```python
from build123d import *

# Parameters (mm, degrees)
HOLE_WIZARD_M3_1_D     = 2.5
HOLE_WIZARD_M3_1_DEPTH = 10
HOLE_WIZARD_M3_2_D     = 2.5
HOLE_WIZARD_M3_2_DEPTH = 9.5
HOLE_WIZARD_M3_2_TIP   = 0.751075774
EXTRUDE_START          = 6
SKETCH_9_R             = 3.5
SKETCH_9_R_2           = 3
EXTRUDE_1_DEPTH        = 6


with BuildPart() as part:
    # 草图1 → 旋转1 (revolve)
    with BuildSketch(Plane.XY, mode=Mode.PRIVATE) as revolve_1_sk:
        Polygon((0, 9), (0, 3), (57.5, 3), (57.5, 8.75), (41.5, 8.75), (41.5, 9), (36.5, 9), (36.5, 6), (10, 6), (10, 9), align=None)
    revolve(revolve_1_sk.sketch.rotate(Axis((0, 0, 0), (1, 0, 0)), 90), axis=Axis((0, 0, 0), (1, 0, 0)))

    # M3 螺纹孔1
    with Locations(Plane.ZY):
        with Locations((0, 6), (6, 0), (0, -6), (-6, 0)):
            Hole(HOLE_WIZARD_M3_1_D / 2, depth=HOLE_WIZARD_M3_1_DEPTH)

    # M3 螺纹孔2
    with Locations(Plane(origin=(57.5, 0, 0), x_dir=(0, 0, -1), z_dir=(1, 0, 0))):
        with Locations((0, 6.25), (6.25, 0), (0, -6.25), (-6.25, 0)):
            Hole(HOLE_WIZARD_M3_2_D / 2, depth=HOLE_WIZARD_M3_2_DEPTH)
            with Locations((0, 0, -(HOLE_WIZARD_M3_2_DEPTH + HOLE_WIZARD_M3_2_TIP / 2))):  # 118° drill point
                Cone(0, HOLE_WIZARD_M3_2_D / 2, HOLE_WIZARD_M3_2_TIP, mode=Mode.SUBTRACT)

    # 草图9 → 凸台-拉伸1 (add)
    with BuildSketch(Plane(origin=(57.5, 0, 0), x_dir=(0, 0, -1), z_dir=(1, 0, 0)).offset(EXTRUDE_START)):
        with Locations(Location((0, 0, 0), (0, 0, 180))):
            Circle(SKETCH_9_R)
        with Locations(Location((0, 0, 0), (0, 0, 180))):
            Circle(SKETCH_9_R_2, mode=Mode.SUBTRACT)
    extrude(amount=-EXTRUDE_1_DEPTH)


solid = part.part
```
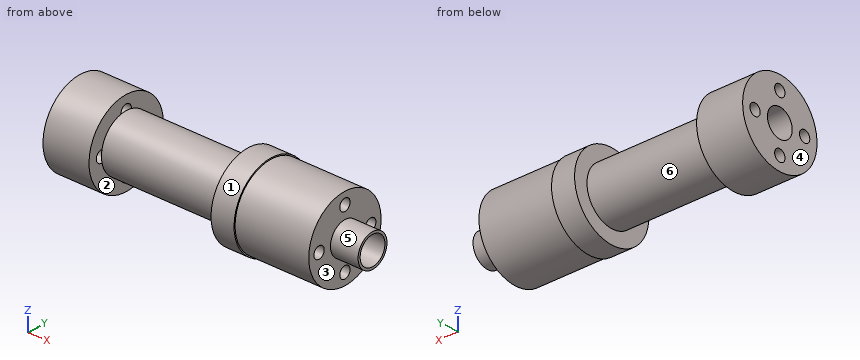
Input: part model. Units: mm. Frame: model coordinates. Face numbers are marked on the shaded views. A direction names the side the tool comes from. Give positions to 0.01 mm unless a question says otherwise; leave off trailing zeros. Order: outer loops, then holes, each group sorted by start corner. A loop starts at its lowest first (then second) coordinate and runs counter-clockwise, first axis right, second up.
1. Cut plane C-C (x = 46). Return loops of the section in (y, z).
Computed:
outline: circle Ø17.5 at (0, 0); hole circle Ø6 at (0, 0)
2. Pin query (flat end, axial travel): pin 1 Ø2 at (y, z) = (0, 6.25) entering from +X; pin 2 Ø4 at (y, z) = (0, -6.25) entering from +X; pin 3 Ø1.4 at (y, z) = (5.5, 0) entering from -X. Return the tip coordinate at first contact, or that it passes through.
Computed:
pin 1: stops at x = 47.85
pin 2: stops at x = 57.5
pin 3: stops at x = 10
3. Draft query along X for the marked faces 4, 5 and 6. Return one class per face: released by +X, released by -X, zero draft, split by the parting line, or undercut.
Computed:
face 4: released by -X
face 5: zero draft
face 6: undercut
4. Cut plane B-B (x = 39). Return loops of the section in (y, z), and give its area (3 significant figures).
Computed:
outline: circle Ø18 at (0, 0); hole circle Ø6 at (0, 0)
area: 226 mm2
5. Line query: probe 1 along Y at (x, z) = (7, 0); probe 2 along X at (y, z) = (-4.75, 7.25); probe 3 along X at (y, z) = (-3.75, 3). Output: solid intervals per line, ascending.
Computed:
probe 1: y = -9 to -7.25, -4.75 to -3, 3 to 4.75, 7.25 to 9
probe 2: x = 0 to 10, 36.5 to 57.5
probe 3: x = 0 to 57.5
6. Set-up query: the marked faces 1, 2 and 3. Return all of +Z, -Z, +X, -X, +Y, -Y with unobstructed straight access to the full face (end or side cutting, diameter ignored); none if empty.
Computed:
face 1: +X, -X
face 2: none
face 3: +X
7. Cut plane A-A (x = 8). Return loops of the section in (y, z), and give its area (3 significant figures).
Computed:
outline: circle Ø18 at (0, 0); hole circle Ø2.5 at (-6, 0); hole circle Ø6 at (0, 0); hole circle Ø2.5 at (0, -6); hole circle Ø2.5 at (0, 6); hole circle Ø2.5 at (6, 0)
area: 207 mm2
